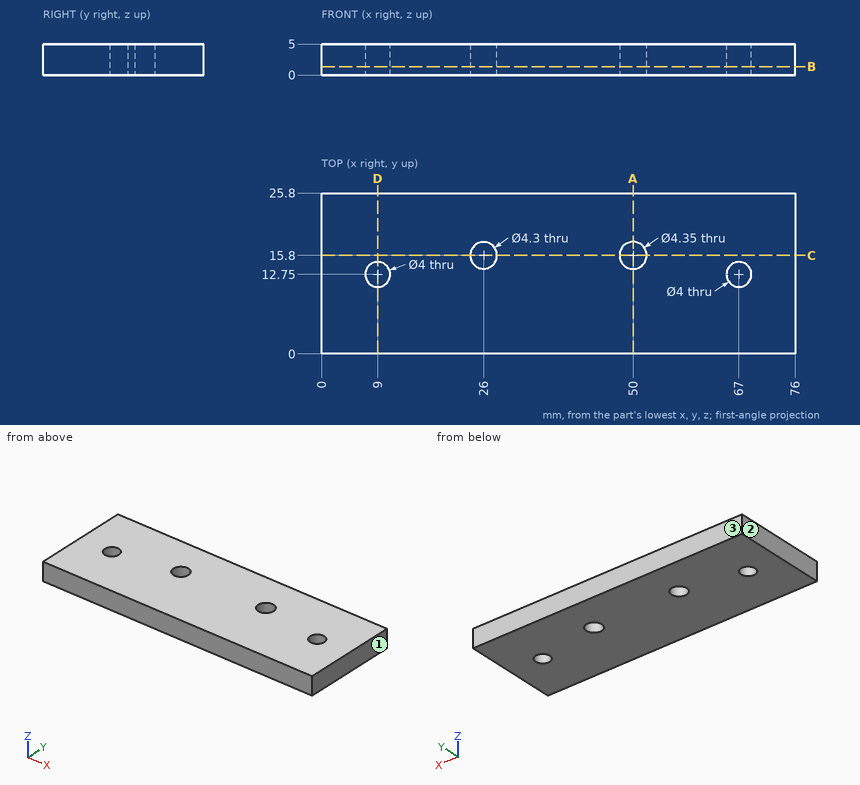
Geometry check sheet. Reference: drawing and pictorial views, mm from the part's lowest x, y, z. Round coordinates to 2 decimals unless told otherwise and drop trailing zeros. Loops run counter-clockwise (first coordinate to the right, second up) from the corner with the lowest first, then second, coordinate; pieces in that order, holes last. Notation, with made-up numbers: (-1, -25) -> (46, -25) arc R13 cw to (46, 0) -> close; hole circle Ø11 at (38, 83.25). An arc over 180 degrees is marked (long way). Answer as a JSON object with one key per item and string values. Group by question number.
Item 1: Cross-section at A-A, the plane x = 50. Record the cut outline in (y, z) (3 decimals).
Item 2: Cross-section at C-C, the plane y = 15.8. Record the cut outline in (x, z) (3 decimals), plus the area to 3 significant figures.
Item 3: Cross-section at D-D, the plane x = 9. Record the cut outline in (y, z).
Item 4: Cross-section at B-B, the plane z = 1.35. Record the cut outline in (x, y) (3 decimals), plus the area to 3 significant figures.
Item 5: Thickness scan on line 1 along Y through (x, z) = (9, 3.95); line 2 along X through (y, z) = (15.75, 0.85); line 3 along X through (y, z) = (12.5, 0.2). Record the ranges inside material, lowest first.
Item 6: Release check for a two-part mould opening along X. For the marked faces 1, 2 and 3 record: pulls with the +X half, pulls with the -X half, needs draft (parallel to the pull), parting line crosses it, or undercut.
Determined:
{
 "1": {"outline": "(0, 0) -> (13.625, 0) -> (13.625, 5) -> (0, 5) -> close; (17.975, 0) -> (25.8, 0) -> (25.8, 5) -> (17.975, 5) -> close"},
 "2": {"outline": "(0, 0) -> (23.85, 0) -> (23.85, 5) -> (0, 5) -> close; (28.15, 0) -> (47.825, 0) -> (47.825, 5) -> (28.15, 5) -> close; (52.175, 0) -> (76, 0) -> (76, 5) -> (52.175, 5) -> close", "area": "337 mm²"},
 "3": {"outline": "(0, 0) -> (10.75, 0) -> (10.75, 5) -> (0, 5) -> close; (14.75, 0) -> (25.8, 0) -> (25.8, 5) -> (14.75, 5) -> close"},
 "4": {"outline": "(0, 0) -> (76, 0) -> (76, 25.8) -> (0, 25.8) -> close; hole circle Ø4 at (9, 12.75); hole circle Ø4.3 at (26, 15.8); hole circle Ø4.35 at (50, 15.8); hole circle Ø4 at (67, 12.75)", "area": "1,910 mm²"},
 "5": {"line 1": "y = 0 to 10.75, 14.75 to 25.8", "line 2": "x = 0 to 23.85, 28.15 to 47.83, 52.17 to 76", "line 3": "x = 0 to 7.02, 10.98 to 65.02, 68.98 to 76"},
 "6": {"face 1": "pulls with the +X half", "face 2": "pulls with the -X half", "face 3": "needs draft"}
}
